CAD build for the part. Positions are in the model's coordinates, mm. A direction names the side the tool comes from. Coordinates: 2 decimals unless noted, no trailing zeros. Write each loop counter-clockwise with the first axis right and the second up, starting at its lowest first coordinate (ties: lowest second). Pieces come first, ordered by that corner, then holes. Notation, with made-up numbers: (24.5, 63.5) -> (48.5, 63.5) arc R23 ccw to (48.5, 85.5) -> close; hole circle Ø11 at (52, 53). An arc over 180 degrees is marked (long way). Answer as CSV lines item,"result".
```python
from build123d import *

# Parameters (mm, degrees)
F0_W      = 609.6
F0_H      = 609.6
F0_R      = 7.540625
F0_R_2    = 5.159375
F1_DEPTH  = 19.05
F2_DEPTH  = 12.7
F3_W      = 609.6
F3_H      = 3.175
F4_DEPTH  = 12.7
F5_R      = 9.525
F6_DEPTH  = 6.35
F7_W      = 25.4
F7_H      = 0.0254
F7_W_2    = 50
F8_DEPTH  = 0.254
F10_DEPTH = 2.54


# Not quite as in the source:
# - a pattern or mirror of a feature is missing from the dataset's text; its kind, count and spacing are read off the source's solid


with BuildPart() as f1:
    # F0 (on Top) → F1 (new body)
    with BuildSketch(Plane.XY):
        Rectangle(F0_W, F0_H)
        with Locations((-271.4625, -269.875)):
            Circle(F0_R, mode=Mode.SUBTRACT)
        with Locations((-292.1, -220.6625)):
            Circle(F0_R_2, mode=Mode.SUBTRACT)
        with Locations((-292.1, -188.9125)):
            Circle(F0_R_2, mode=Mode.SUBTRACT)
        with Locations((-227.80625, -220.6625)):
            Circle(F0_R_2, mode=Mode.SUBTRACT)
        with Locations((-227.80625, -188.9125)):
            Circle(F0_R_2, mode=Mode.SUBTRACT)
        with Locations((-292.1, 206.375)):
            Circle(F0_R_2, mode=Mode.SUBTRACT)
        with Locations((-227.80625, 206.375)):
            Circle(F0_R_2, mode=Mode.SUBTRACT)
        with Locations((-292.1, 238.125)):
            Circle(F0_R_2, mode=Mode.SUBTRACT)
        with Locations((-271.4625, 254)):
            Circle(F0_R, mode=Mode.SUBTRACT)
        with Locations((-227.80625, 238.125)):
            Circle(F0_R_2, mode=Mode.SUBTRACT)
        with Locations((-271.4625, 254)):
            Circle(F0_R)
        with Locations((-292.1, 238.125)):
            Circle(F0_R_2)
        with Locations((-292.1, 206.375)):
            Circle(F0_R_2)
        with Locations((-227.80625, 206.375)):
            Circle(F0_R_2)
        with Locations((-227.80625, 238.125)):
            Circle(F0_R_2)
        with Locations((-227.80625, -188.9125)):
            Circle(F0_R_2)
        with Locations((-227.80625, -220.6625)):
            Circle(F0_R_2)
        with Locations((-292.1, -220.6625)):
            Circle(F0_R_2)
        with Locations((-292.1, -188.9125)):
            Circle(F0_R_2)
        with Locations((-271.4625, -269.875)):
            Circle(F0_R)
    extrude(amount=-F1_DEPTH)

    # F0 (on Top) → F2 (cut)
    with BuildSketch(Plane.XY):
        with Locations((-271.4625, -269.875)):
            Circle(F0_R)
        with Locations((-292.1, -220.6625)):
            Circle(F0_R_2)
        with Locations((-227.80625, -220.6625)):
            Circle(F0_R_2)
        with Locations((-227.80625, -188.9125)):
            Circle(F0_R_2)
        with Locations((-292.1, -188.9125)):
            Circle(F0_R_2)
        with Locations((-292.1, 206.375)):
            Circle(F0_R_2)
        with Locations((-227.80625, 206.375)):
            Circle(F0_R_2)
        with Locations((-227.80625, 238.125)):
            Circle(F0_R_2)
        with Locations((-292.1, 238.125)):
            Circle(F0_R_2)
        with Locations((-271.4625, 254)):
            Circle(F0_R)
    f2 = extrude(amount=-F2_DEPTH, mode=Mode.SUBTRACT)

    # F2_copies: F2 across plane
    add(f2.mirror(Plane(origin=(0, 0, 0), x_dir=(0, 0, 1), z_dir=(1, 0, 0))), mode=Mode.SUBTRACT)

    # F3 (on face) → F4 (cut)
    with BuildSketch(Plane(origin=(0, 0, -19.05), x_dir=(1, 0, 0), z_dir=(0, 0, -1))):
        with Locations((0, -293.6875)):
            Rectangle(F3_W, F3_H)
    extrude(amount=-F4_DEPTH, mode=Mode.SUBTRACT)

    # F5 (on face) → F6 (cut)
    with BuildSketch(Plane(origin=(0, 0, -19.05), x_dir=(1, 0, 0), z_dir=(0, 0, -1))):
        with Locations((260.35, -274.6375)):
            Circle(F5_R)
        with Locations((204.7875, -274.6375)):
            Circle(F5_R)
        with Locations((204.7875, -232.56875)):
            Circle(F5_R)
        with Locations((260.35, -232.56875)):
            Circle(F5_R)
        with Locations((-204.7875, -274.6375)):
            Circle(F5_R)
        with Locations((-260.35, -274.6375)):
            Circle(F5_R)
        with Locations((-260.35, -232.56875)):
            Circle(F5_R)
        with Locations((-204.7875, -232.56875)):
            Circle(F5_R)
        with Locations((-204.7875, 205.58125)):
            Circle(F5_R)
        with Locations((-260.35, 205.58125)):
            Circle(F5_R)
        with Locations((-260.35, 247.65)):
            Circle(F5_R)
        with Locations((-204.7875, 247.65)):
            Circle(F5_R)
        with Locations((204.7875, 247.65)):
            Circle(F5_R)
        with Locations((204.7875, 205.58125)):
            Circle(F5_R)
        with Locations((260.35, 205.58125)):
            Circle(F5_R)
        with Locations((260.35, 247.65)):
            Circle(F5_R)
    extrude(amount=-F6_DEPTH, mode=Mode.SUBTRACT)

    # F7 (on face) → F8 (cut)
    with BuildSketch(Plane(origin=(0, 0, -19.05), x_dir=(1, 0, 0), z_dir=(0, 0, -1))):
        with Locations((-156.0546457767, -265.0721735465)):
            Rectangle(F7_W, F7_H)
        with Locations((-145.1898425817, -234.882380328)):
            Rectangle(F7_W_2, F7_H)
    extrude(amount=-F8_DEPTH, mode=Mode.SUBTRACT)

    # F9 (on face) → F10 (cut)
    with BuildSketch(Plane.XY):
        with BuildLine():
            Line((-273.0246, 304.8), (-273.05, 304.8))
            Line((-273.05, 304.8), (-273.05, 261.3716259496))
            ThreePointArc((-273.05, 261.3716259496), (-273.0373023354, 261.3743489879), (-273.0246, 261.3770501544))
            Line((-273.0246, 261.3770501544), (-273.0246, 304.8))
        make_face()
        with BuildLine():
            ThreePointArc((-273.0246, 261.3770501544), (-273.0373023354, 261.3743489879), (-273.05, 261.3716259496))
            Line((-273.05, 261.3716259496), (-273.05, 246.6283740504))
            ThreePointArc((-273.05, 246.6283740504), (-273.0373023354, 246.6256510121), (-273.0246, 246.6229498456))
            Line((-273.0246, 246.6229498456), (-273.0246, 261.3770501544))
        make_face()
        with BuildLine():
            Line((273.05, 304.8), (273.0246, 304.8))
            Line((273.0246, 304.8), (273.0246, 261.3770501544))
            ThreePointArc((273.0246, 261.3770501544), (273.0373023354, 261.3743489879), (273.05, 261.3716259496))
            Line((273.05, 261.3716259496), (273.05, 304.8))
        make_face()
        with BuildLine():
            ThreePointArc((-273.0246, 246.6229498456), (-273.0373023354, 246.6256510121), (-273.05, 246.6283740504))
            Line((-273.05, 246.6283740504), (-273.05, -262.5033740504))
            ThreePointArc((-273.05, -262.5033740504), (-273.0373023354, -262.5006510121), (-273.0246, -262.4979498456))
            Line((-273.0246, -262.4979498456), (-273.0246, 246.6229498456))
        make_face()
        with BuildLine():
            ThreePointArc((-273.0246, -262.4979498456), (-273.0373023354, -262.5006510121), (-273.05, -262.5033740504))
            Line((-273.05, -262.5033740504), (-273.05, -277.2466259496))
            ThreePointArc((-273.05, -277.2466259496), (-273.0373023354, -277.2493489879), (-273.0246, -277.2520501544))
            Line((-273.0246, -277.2520501544), (-273.0246, -262.4979498456))
        make_face()
        with BuildLine():
            Line((-273.05, -277.2466259496), (-273.05, -304.8))
            Line((-273.05, -304.8), (-273.0246, -304.8))
            Line((-273.0246, -304.8), (-273.0246, -277.2520501544))
            ThreePointArc((-273.0246, -277.2520501544), (-273.0373023354, -277.2493489879), (-273.05, -277.2466259496))
        make_face()
        with BuildLine():
            ThreePointArc((273.05, 246.6283740504), (273.0373023354, 246.6256510121), (273.0246, 246.6229498456))
            Line((273.0246, 246.6229498456), (273.0246, -262.4979498456))
            ThreePointArc((273.0246, -262.4979498456), (273.0373023354, -262.5006510121), (273.05, -262.5033740504))
            Line((273.05, -262.5033740504), (273.05, 246.6283740504))
        make_face()
        with BuildLine():
            Line((273.0246, -277.2520501544), (273.0246, -304.8))
            Line((273.0246, -304.8), (273.05, -304.8))
            Line((273.05, -304.8), (273.05, -277.2466259496))
            ThreePointArc((273.05, -277.2466259496), (273.0373023354, -277.2493489879), (273.0246, -277.2520501544))
        make_face()
    extrude(amount=-F10_DEPTH, mode=Mode.SUBTRACT)


solid = f1.part
```
Item 1: Saw through at A-A on y = 254. Give the cut face in (x, z).
Answer below:
outline,"(-304.8, -19.05) -> (304.8, -19.05) -> (304.8, 0) -> (279, 0) -> (279, -12.7) -> (263.92, -12.7) -> (263.92, 0) -> (-263.92, 0) -> (-263.92, -12.7) -> (-279, -12.7) -> (-279, 0) -> (-304.8, 0) -> close"
Item 2: Wall check: line 1 (Y direction, x = -259.5, z = -17.75) (1 decimal); line 2 (Y direction, x = 292.1, z = -6.25); line 3 (Y direction, x = 273.5, z = -10.5) (3 decimals). Give the ranges that are in metal, low to high. Write a range as from..to.
Answer below:
line 1,"y = -304.8..-257.1, -238.2..-215.1, -196.1..223.1, 242.1..265.2, 284.1..292.1, 295.3..304.8"
line 2,"y = -304.8..-225.82, -215.5..-194.07, -183.75..201.22, 211.53..232.97, 243.28..304.8"
line 3,"y = -304.8..-277.135, -262.615..246.74, 261.26..292.1, 295.275..304.8"
Item 3: Two-plate mould, pull along X, no slides. Class faces 4 (the flat face through (-304.8, -4, -9)), 5 (the flat face through (205, -206, -12.7)), 6 (the flat face through (-4, -304.8, -9)): pulls with the +X half, pulls with the -X half, needs draft (parallel to the pull), parting line crosses it, or undercut.
Answer below:
face 4,"pulls with the -X half"
face 5,"undercut"
face 6,"needs draft"
Item 4: 3-axis set-ups, long thin cutter, end or side, ignore diameter. For faces 1 (the flat face through (-4, 304.8, -9)), 2 (the cylindrical face through (-267.909, -241.854, -15.919)), 3 (the cylindrical face through (278.996, 254.332, -6.261)): which of +Z, -Z, +X, -X, +Y, -Y reach the whole face in a straight line?
Answer below:
face 1,"+Z, -Z, +X, -X, +Y"
face 2,"-Z"
face 3,"+Z"
Item 5: Flat gauge pin, fed straight in: pin 1 (3 mm diameter, centred on x = 226, y = -187, fed in from +Z). Where does the tip first touch, or does it go through?
Answer below:
pin 1,"stops at z = -12.7"
